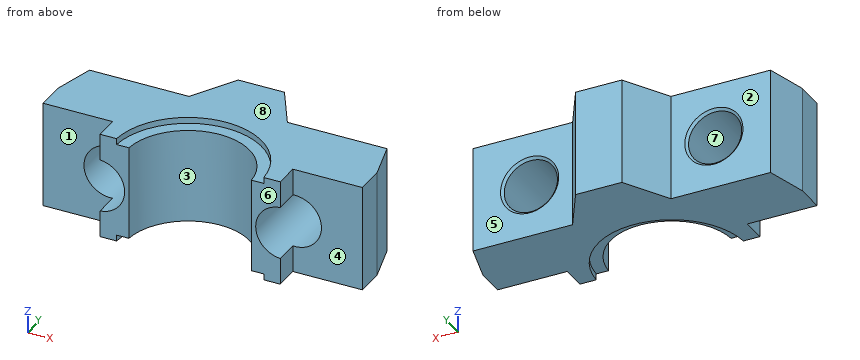
from build123d import *

# Parameters (mm, degrees)
EXTRUDE_1_DEPTH     = 26
SKETCH_2_R          = 15
CUT_EXTRUDE_1_DEPTH = 59.497863209
SKETCH_3_R          = 18
CUT_EXTRUDE_2_DEPTH = 1.5
CUT_EXTRUDE_START   = -1.5
SKETCH_4_R          = 18
CUT_EXTRUDE_3_DEPTH = 1.5
EXTRUDE_2_DEPTH     = 26
SKETCH_6_R          = 6.5
CUT_EXTRUDE_5_DEPTH = 53.211109929
CHAMFER_1_SIZE      = 0.6


with BuildPart() as part:
    # Эскиз1 → Бобышка-Вытянуть1 (new body)
    with BuildSketch(Plane.XY):
        with BuildLine():
            Line((-35.09985755, 24), (-12, 24))
            Line((-12, 24), (-5.649147039, 35))
            Line((-5.649147039, 35), (5.649147039, 35))
            Line((5.649147039, 35), (12, 24))
            Line((12, 24), (35.09985755, 24))
            ThreePointArc((35.09985755, 24), (38.012461407, 15.720824375), (39, 7))
            Line((39, 7), (22, 7))
            Line((22, 7), (22, 1))
            Line((22, 1), (-22, 1))
            Line((-22, 1), (-22, 7))
            Line((-22, 7), (-39, 7))
            ThreePointArc((-39, 7), (-38.012461407, 15.720824375), (-35.09985755, 24))
        make_face()
    extrude(amount=-EXTRUDE_1_DEPTH)

    # Эскиз2 → Вырез-Вытянуть1 (cut, through all)
    with BuildSketch(Plane.XY):
        Circle(SKETCH_2_R)
    extrude(amount=-CUT_EXTRUDE_1_DEPTH, mode=Mode.SUBTRACT)

    # Эскиз3 → Вырез-Вытянуть2 (cut)
    with BuildSketch(Plane.XY):
        Circle(SKETCH_3_R)
    extrude(amount=-CUT_EXTRUDE_2_DEPTH, mode=Mode.SUBTRACT)

    # Эскиз4 → Вырез-Вытянуть3 (cut)
    with BuildSketch(Plane(origin=(0, 0, -26), x_dir=(-1, 0, 0), z_dir=(0, 0, -1)).offset(CUT_EXTRUDE_START)):
        Circle(SKETCH_4_R)
    extrude(amount=CUT_EXTRUDE_3_DEPTH, mode=Mode.SUBTRACT)

    # Эскиз9 → Бобышка-Вытянуть2 (add)
    with BuildSketch(Plane.XY):
        Polygon((-39, 7), (-39, 14), (-36.320508076, 24), (-22, 24), (-22, 7), align=None)
        Polygon((39, 7), (39, 14), (36.320508076, 24), (22, 24), (22, 7), align=None)
    extrude(amount=-EXTRUDE_2_DEPTH)

    # Эскиз6 → Вырез-Вытянуть5 (cut, through all)
    with BuildSketch(Plane(origin=(0, 24, 0), x_dir=(1, 0, 0), z_dir=(0, 1, 0))):
        with Locations(Location((-22.5, 13, 0), (0, 0, 270))):
            Circle(SKETCH_6_R)
        with Locations(Location((22.5, 13, 0), (0, 0, 270))):
            Circle(SKETCH_6_R)
    extrude(amount=-CUT_EXTRUDE_5_DEPTH, mode=Mode.SUBTRACT)

    # Фаска1
    chamfer_1_edges = [part.edges().sort_by_distance(p)[0] for p in [
        (-22.5, 24, -19.5),
        (22.5, 24, -19.5),
    ]]
    chamfer(chamfer_1_edges, length=CHAMFER_1_SIZE)


solid = part.part
Design review of the part built by this model. Coordinates are the model's own, in mm. Face numbers are marked on the shaded views. A direction names the side the tool comes from. Give positions to 0.01 mm unless a question says otherwise; leave off trailing zeros. Write each loop counter-clockwise with the first axis right and the second up, starting at its lowest first coordinate (ties: lowest second). Pieces come first, ordered by that corner, then holes. Notation, with made-up numbers: M -33.75,61 L 25.25,61 A22 cw 25.25,89 Z; hole C 53,56.25 d6. An arc over 180 degrees is marked long. Answer as a JSON object with one key per item and string values. Group by question number.
1) For line 1 along X through (y, z) = (17.25, -13); line 2 along X through (y, z) = (11.5, -14.25); line 3 along X through (y, z) = (19, -13), list the stretches that pass through material, from the lowest coordinate up.
2) Clearance check with flat-ended pins moving along their axes: pin 1 Ø1.8 at (y, z) = (4.5, -4) entering from -X; pin 2 Ø8.5 at (x, z) = (33, -8.5) entering from -Y; pin 3 Ø3 at (y, z) = (3, -23) entering from +X; pin 4 Ø13.5 at (x, y) = (-6.5, 13) entering from -Z. State where each tip first meets the part, or that it passes through.
3) Tool access review of the marked faces 1, 2, 3, 4 and 5: name each direction out of +Z, -Z, +X, -X, +Y, -Y from which nothing blocks a thin tool from reaching the whole face with its end or side.
4) We need section D-D (y = 5). Give the boundary of the cut face in (x, z).
5) Mouldability with a two-part tool opening along Z and no side actions: class the marked faces 6, 7 and 8 as released by +Z, released by -Z, zero draft, split by the parting line, or undercut.
6) We need section C-C (z = -22). Give the boundary of the cut face in (x, y), and give its area (3 significant figures).
7) We need section B-B (y = 13). Give the boundary of the cut face in (x, z).
8) We need section A-A (z = -13). Give the boundary of the cut face in (x, y).
Answer key:
{
 "1": {"line 1": "x = -38.13 to -29, -16 to 16, 29 to 38.13", "line 2": "x = -39 to -28.88, -16.12 to -9.63, 9.63 to 16.12, 28.88 to 39", "line 3": "x = -37.66 to -29, -16 to 16, 29 to 37.66"},
 "2": {"pin 1": "stops at x = -22", "pin 2": "stops at y = 7", "pin 3": "stops at x = 22", "pin 4": "stops at z = -26"},
 "3": {"face 1": "+Z, -Z, -X, -Y", "face 2": "+Z, -Z, -X, +Y", "face 3": "+Z, -Z, -Y", "face 4": "+Z, -Z, +X, -Y", "face 5": "+Z, -Z, +X, +Y"},
 "4": {"outline": "M -22,-26 L -17.29,-26 L -17.29,-24.5 L -14.14,-24.5 L -14.14,-1.5 L -17.29,-1.5 L -17.29,0 L -22,0 L -22,-6.52 A6.5 cw -22,-19.48 Z; M 14.14,-24.5 L 17.29,-24.5 L 17.29,-26 L 22,-26 L 22,-19.48 A6.5 cw 22,-6.52 L 22,0 L 17.29,0 L 17.29,-1.5 L 14.14,-1.5 Z"},
 "5": {"face 6": "zero draft", "face 7": "undercut", "face 8": "released by +Z"},
 "6": {"outline": "M -39,7 L -22,7 L -22,1 L -14.97,1 A15 cw 14.97,1 L 22,1 L 22,7 L 39,7 L 39,14 L 36.32,24 L 12,24 L 5.65,35 L -5.65,35 L -12,24 L -36.32,24 L -39,14 Z", "area": "1,430 mm²"},
 "7": {"outline": "M -39,-26 L -12.45,-26 L -12.45,-24.5 L -7.48,-24.5 L -7.48,-1.5 L -12.45,-1.5 L -12.45,0 L -39,0 Z; M 7.48,-24.5 L 12.45,-24.5 L 12.45,-26 L 39,-26 L 39,0 L 12.45,0 L 12.45,-1.5 L 7.48,-1.5 Z; hole C -22.5,-13 d13; hole C 22.5,-13 d13"},
 "8": {"outline": "M -39,7 L -29,7 L -29,23.4 L -29.6,24 L -36.32,24 L -39,14 Z; M -16,1 L -14.97,1 A15 cw 14.97,1 L 16,1 L 16,23.4 L 15.4,24 L 12,24 L 5.65,35 L -5.65,35 L -12,24 L -15.4,24 L -16,23.4 Z; M 29,7 L 39,7 L 39,14 L 36.32,24 L 29.6,24 L 29,23.4 Z"}
}
